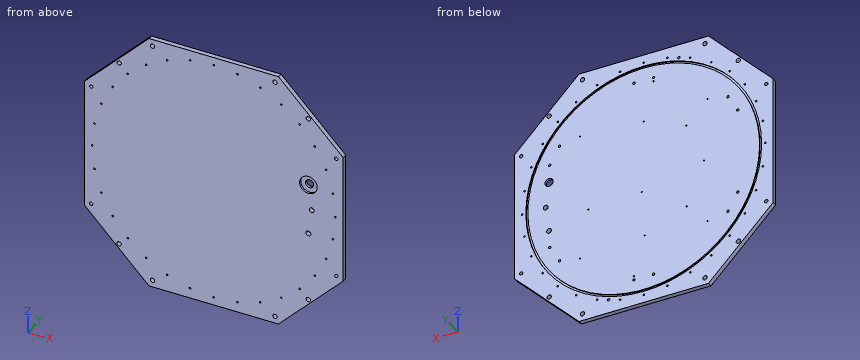
from build123d import *

# Parameters (mm, degrees)
BASE_PLATE_PROFILE_DEPTH                     = 4.7625
M3_CLEARANCE_HOLE_FOR_CYLINDER_D             = 3.4
M6X1_TAPPED_HOLE_FOR_SUPPORT_PILLARS_D       = 5
M6X1_TAPPED_HOLE_FOR_SUPPORT_PILLARS_DEPTH   = 6
M6X1_TAPPED_HOLE_FOR_SUPPORT_PILLARS_TIP     = 1.502151548
F_3_0MM_DOWEL_HOLE_FOR_SUPPORT_PILLARS_D     = 3
F_3_0MM_DOWEL_HOLE_FOR_SUPPORT_PILLARS_DEPTH = 6
F_3_0MM_DOWEL_HOLE_FOR_SUPPORT_PILLARS_TIP   = 0.901290929
M3X0_5_TAPPED_HOLE_FOR_PCB_STANDOFFS_D       = 2.5
M3X0_5_TAPPED_HOLE_FOR_PCB_STANDOFFS_DEPTH   = 6.5
M3X0_5_TAPPED_HOLE_FOR_PCB_STANDOFFS_TIP     = 0.751075774
M8_CLEARANCE_HOLE_FOR_LIFTING_ALIGNM_D       = 9
M8X1_25_TAPPED_HOLE_FOR_SUPER_STRUCTURE_D    = 6.8
F_7_16_20_TAPPED_HOLE_FOR_PENETRATOR_D       = 9.92124
SKETCH28_R                                   = 240.5
SKETCH28_R_2                                 = 236.3344
O_RING_GROOVE_DEPTH                          = 2.413
CIRPATTERN_EXTRACABLES_COUNT                 = 2
CIRPATTERN_EXTRACABLES_ANGLE                 = 15
F_5_8_CLEARANCE_HOLE1_D                      = 16.66748
SKETCH35_R                                   = 18
CUT_EXTRUDE1_DEPTH                           = 4.5
M8_CLEARANCE_HOLE_D                          = 9
F_5_0MM_DOWEL_HOLE1_D                        = 5.05
F_5_0MM_DOWEL_HOLE1_DEPTH                    = 5
F_5_0MM_DOWEL_HOLE1_TIP                      = 1.517173063


with BuildPart() as part:
    # Sketch1 → Base Plate Profile (new, symmetric)
    with BuildSketch(Plane(origin=(0, 0, 0), x_dir=(1, 0, 0), z_dir=(0, 1, 0))):
        Polygon((-131.979797464, 264), (131.979797464, 264), (264, 131.979797464), (264, -131.979797464), (131.979797464, -264), (-131.979797464, -264), (-264, -131.979797464), (-264, 131.979797464), align=None)
    extrude(amount=BASE_PLATE_PROFILE_DEPTH, both=True)

    # M3 Clearance Hole - For Cylinder (through all)
    with Locations(Plane(origin=(0, 4.7625, 0), x_dir=(1, 0, 0), z_dir=(0, 1, 0))):
        with Locations((248, 0), (243.23474954, -48.38239986), (229.122124063, -94.905491227), (206.204463851, -137.781417789), (175.362481734, -175.362481734), (137.781417789, -206.204463851), (94.905491227, -229.122124063), (48.38239986, -243.23474954), (0, -248), (-48.38239986, -243.23474954), (-94.905491227, -229.122124063), (-137.781417789, -206.204463851), (-175.362481734, -175.362481734), (-206.204463851, -137.781417789), (-229.122124063, -94.905491227), (-243.23474954, -48.38239986), (-248, 0), (-243.23474954, 48.38239986), (-229.122124063, 94.905491227), (-206.204463851, 137.781417789), (-175.362481734, 175.362481734), (-137.781417789, 206.204463851), (-94.905491227, 229.122124063), (-48.38239986, 243.23474954), (0, 248), (48.38239986, 243.23474954), (94.905491227, 229.122124063), (137.781417789, 206.204463851), (175.362481734, 175.362481734), (206.204463851, 137.781417789), (229.122124063, 94.905491227), (243.23474954, 48.38239986)):
            Hole(M3_CLEARANCE_HOLE_FOR_CYLINDER_D / 2)

    # M6x1 Tapped Hole - For Support Pillars
    with Locations(Plane(origin=(0, 4.7625, 0), x_dir=(1, 0, 0), z_dir=(0, 1, 0))):
        with Locations((-20, 210), (20, 210), (171.865334795, 122.320508076), (191.865334795, 87.679491924), (191.865334795, -87.679491924), (171.865334795, -122.320508076), (20, -210), (-20, -210), (-171.865334795, -122.320508076), (-191.865334795, -87.679491924), (-191.865334795, 87.679491924), (-171.865334795, 122.320508076)):
            Hole(M6X1_TAPPED_HOLE_FOR_SUPPORT_PILLARS_D / 2, depth=M6X1_TAPPED_HOLE_FOR_SUPPORT_PILLARS_DEPTH)
            with Locations((0, 0, -(M6X1_TAPPED_HOLE_FOR_SUPPORT_PILLARS_DEPTH + M6X1_TAPPED_HOLE_FOR_SUPPORT_PILLARS_TIP / 2))):  # 118° drill point
                Cone(0, M6X1_TAPPED_HOLE_FOR_SUPPORT_PILLARS_D / 2, M6X1_TAPPED_HOLE_FOR_SUPPORT_PILLARS_TIP, mode=Mode.SUBTRACT)

    # Ø3.0mm Dowel Hole - For Support Pillars
    with Locations(Plane(origin=(0, 4.7625, 0), x_dir=(1, 0, 0), z_dir=(0, 1, 0))):
        with Locations((20, 202), (-20, -202)):
            Hole(F_3_0MM_DOWEL_HOLE_FOR_SUPPORT_PILLARS_D / 2, depth=F_3_0MM_DOWEL_HOLE_FOR_SUPPORT_PILLARS_DEPTH)
            with Locations((0, 0, -(F_3_0MM_DOWEL_HOLE_FOR_SUPPORT_PILLARS_DEPTH + F_3_0MM_DOWEL_HOLE_FOR_SUPPORT_PILLARS_TIP / 2))):  # 118° drill point
                Cone(0, F_3_0MM_DOWEL_HOLE_FOR_SUPPORT_PILLARS_D / 2, F_3_0MM_DOWEL_HOLE_FOR_SUPPORT_PILLARS_TIP, mode=Mode.SUBTRACT)

    # M3x0.5 Tapped Hole - For PCB Standoffs
    with Locations(Plane(origin=(0, 4.7625, 0), x_dir=(1, 0, 0), z_dir=(0, 1, 0))):
        with Locations((113, 31), (-130, -130), (130, -130), (130, 130), (-130, 130), (-86.8, -86.7), (0, -122), (-123, -1), (-87.7, 85.8), (4, 27), (-2, 122)):
            Hole(M3X0_5_TAPPED_HOLE_FOR_PCB_STANDOFFS_D / 2, depth=M3X0_5_TAPPED_HOLE_FOR_PCB_STANDOFFS_DEPTH)
            with Locations((0, 0, -(M3X0_5_TAPPED_HOLE_FOR_PCB_STANDOFFS_DEPTH + M3X0_5_TAPPED_HOLE_FOR_PCB_STANDOFFS_TIP / 2))):  # 118° drill point
                Cone(0, M3X0_5_TAPPED_HOLE_FOR_PCB_STANDOFFS_D / 2, M3X0_5_TAPPED_HOLE_FOR_PCB_STANDOFFS_TIP, mode=Mode.SUBTRACT)

    # M8 Clearance Hole - For Lifting / Alignment (through all)
    with Locations(Plane(origin=(0, 4.7625, 0), x_dir=(1, 0, 0), z_dir=(0, 1, 0))):
        with Locations((-193.040151264, -193.040151264), (-193.040151264, 193.040151264), (193.040151264, 193.040151264), (193.040151264, -193.040151264)):
            Hole(M8_CLEARANCE_HOLE_FOR_LIFTING_ALIGNM_D / 2)

    # M8x1.25 Tapped Hole -For Super Structure (through all)
    with Locations(Plane(origin=(0, 4.7625, 0), x_dir=(1, 0, 0), z_dir=(0, 1, 0))):
        with Locations((250, 125), (-250, -125), (-250, 125), (250, -125)):
            Hole(M8X1_25_TAPPED_HOLE_FOR_SUPER_STRUCTURE_D / 2)

    # 7/16-20 Tapped Hole - For Penetrator (through all)
    with Locations(Plane(origin=(0, -4.7625, 0), x_dir=(-1, 0, 0), z_dir=(0, -1, 0))):
        with Locations((-200, 0)):
            f_7_16_20_tapped_hole_for_penetrator = Hole(F_7_16_20_TAPPED_HOLE_FOR_PENETRATOR_D / 2)

    # Sketch28 → O-ring Groove (cut)
    with BuildSketch(Plane(origin=(0, 4.7625, 0), x_dir=(1, 0, 0), z_dir=(0, 1, 0))):
        with Locations(Location((0, 0, 0), (0, 0, 270))):
            Circle(SKETCH28_R)
        with Locations(Location((0, 0, 0), (0, 0, 270))):
            Circle(SKETCH28_R_2, mode=Mode.SUBTRACT)
    extrude(amount=-O_RING_GROOVE_DEPTH, mode=Mode.SUBTRACT)

    # CirPattern_extraCables: 7/16-20 Tapped Hole - For Penetrator ×2 about axis
    cirpattern_extracables_axis = Axis((0, -5.23875, 0), (0, 1, 0))
    for i in range(1, CIRPATTERN_EXTRACABLES_COUNT):
        add(f_7_16_20_tapped_hole_for_penetrator.rotate(cirpattern_extracables_axis, i * CIRPATTERN_EXTRACABLES_ANGLE / (CIRPATTERN_EXTRACABLES_COUNT - 1)), mode=Mode.SUBTRACT)

    # 5/8 Clearance Hole1 (through all)
    with Locations(Plane(origin=(0, 4.7625, 0), x_dir=(1, 0, 0), z_dir=(0, 1, 0))):
        with Locations((193.185165258, -51.763809021)):
            Hole(F_5_8_CLEARANCE_HOLE1_D / 2)

    # Sketch35 → Cut-Extrude1 (cut)
    with BuildSketch(Plane.XZ.offset(4.7625)):
        with Locations(Location((193.185165258, 51.763809021, 0), (0, 0, 270))):
            Circle(SKETCH35_R)
    extrude(amount=-CUT_EXTRUDE1_DEPTH, mode=Mode.SUBTRACT)

    # M8 Clearance Hole (through all)
    with Locations(Plane(origin=(-28.123925909, 4.7625, -48.06749493), x_dir=(1, 0, 0), z_dir=(0, 1, 0))):
        with Locations((-96.876074091, -298.06749493), (-96.876074091, 201.93250507), (153.123925909, -298.06749493), (153.123925909, 201.93250507)):
            Hole(M8_CLEARANCE_HOLE_D / 2)

    # Ø5.0mm Dowel Hole1
    with Locations(Plane(origin=(0, 4.7625, 0), x_dir=(1, 0, 0), z_dir=(0, 1, 0))):
        with Locations((71.700315282, 236.364262926), (-71.700315282, -236.364262926)):
            Hole(F_5_0MM_DOWEL_HOLE1_D / 2, depth=F_5_0MM_DOWEL_HOLE1_DEPTH)
            with Locations((0, 0, -(F_5_0MM_DOWEL_HOLE1_DEPTH + F_5_0MM_DOWEL_HOLE1_TIP / 2))):  # 118° drill point
                Cone(0, F_5_0MM_DOWEL_HOLE1_D / 2, F_5_0MM_DOWEL_HOLE1_TIP, mode=Mode.SUBTRACT)


solid = part.part
Read the model definition and answer for the solid it produces. Units are mm, in the model's axes. Round coordinates to 2 decimals unless told otherwise and drop trailing zeros. Loops run counter-clockwise (first coordinate to the right, second up) from the corner with the lowest first, then second, coordinate; pieces in that order, holes last.
Q1. Section A-A on x = -153 is taken. Write down the section's boundary in (y, z).
Q2. Each of these flat-tipped pins is pushed along its axis until it touches: pin 1 (4.5 mm diameter, centred on x = 0, z = -248, fed in from -Y); pin 2 (2 mm diameter, centred on x = 130, z = 130, fed in from +Y); pin 3 (19 mm diameter, centred on x = 193.19, z = 51.76, fed in from -Y). Where does it stop, or does it pass through?
Q3. Consider probe 1 along Z at (x, y) = (-125, 1); probe 2 along X at (y, z) = (0, -125); probe 3 along X at (y, z) = (2.5, -22.5). Determine where each line is inside the solid, lowest interval first.
Output:
1. outline: (-4.76, -242.98) - (4.76, -242.98) - (4.76, -185.56) - (2.35, -185.56) - (2.35, -180.12) - (4.76, -180.12) - (4.76, 180.12) - (2.35, 180.12) - (2.35, 185.56) - (4.76, 185.56) - (4.76, 242.98) - (-4.76, 242.98) - close
2. pin 1: stops at y = -4.76
2. pin 2: stops at y = -1.89
2. pin 3: stops at y = -0.26
3. probe 1: z = -264 to -254.5, -245.5 to 245.5, 254.5 to 264
3. probe 2: x = -264 to -253.4, -246.6 to 246.6, 253.4 to 264
3. probe 3: x = -264 to -239.45, -235.26 to 235.26, 239.45 to 264
